Input: part model. Units: mm. Frame: model coordinates. A direction names the side the tool comes from. Coordinates: 2 decimals unless noted, no trailing zeros. Loops run counter-clockwise (first coordinate to the right, second up) from the corner with the lowest first, then second, coordinate; pieces in that order, holes last. Notation, with made-up numbers: (67, 2.5) -> (121, 2.5) arc R29 ccw to (121, 38.5) -> close; hole circle Ø8 at (-33.5, -5.5). An arc over 180 degrees is marked (long way). Answer as a JSON object with one key per item and string values.
from build123d import *

# Parameters (mm, degrees)
ESQUISSE1_R      = 21.5
EXTRUSION1_DEPTH = 30
ESQUISSE2_R      = 10
EXTRUSION2_DEPTH = 5
ESQUISSE3_R      = 4
EXTRUSION3_DEPTH = 20
ESQUISSE4_R      = 17
EXTRUSION4_DEPTH = 40
ESQUISSE5_R      = 4
EXTRUSION5_DEPTH = 1


with BuildPart() as part:
    # Esquisse1 → Extrusion1 (new body)
    with BuildSketch(Plane.XY):
        Circle(ESQUISSE1_R)
    extrude(amount=EXTRUSION1_DEPTH)

    # Esquisse2 → Extrusion2 (add)
    with BuildSketch(Plane.XY.offset(30)):
        Circle(ESQUISSE2_R)
    extrude(amount=EXTRUSION2_DEPTH)

    # Esquisse3 → Extrusion3 (add)
    with BuildSketch(Plane.XY.offset(35)):
        Circle(ESQUISSE3_R)
    extrude(amount=EXTRUSION3_DEPTH)

    # Esquisse4 → Extrusion4 (add)
    with BuildSketch(Plane(origin=(0, 0, 0), x_dir=(-1, 0, 0), z_dir=(0, 0, -1))):
        with Locations(Location((0, 0, 0), (0, 0, 180))):
            Circle(ESQUISSE4_R)
    extrude(amount=EXTRUSION4_DEPTH)

    # Esquisse5 → Extrusion5 (add)
    with BuildSketch(Plane.XY.offset(30)):
        with Locations(Location((0, 17.5, 0), (0, 0, 89.999550935))):
            Circle(ESQUISSE5_R)
        with Locations(Location((-15.155444566, -8.75, 0), (0, 0, 209.999550935))):
            Circle(ESQUISSE5_R)
        with Locations(Location((15.155444566, -8.75, 0), (0, 0, 329.999550935))):
            Circle(ESQUISSE5_R)
    extrude(amount=EXTRUSION5_DEPTH)


solid = part.part
1. Line query: line 1 along Z through (x, y) = (-11, 10.5); line 2 along Z through (x, y) = (11, -16.5); line 3 along Y through (x, z) = (-14, -32). Output: solid intervals per line, ascending.
Reply:
{"line 1": "z = -40 to 30", "line 2": "z = 0 to 30", "line 3": "y = -9.64 to 9.64"}
2. Section query A-A (y = 0). Return loops of the section in (x, z).
Reply:
{"outline": "(-21.5, 0) -> (-17, 0) -> (-17, -40) -> (17, -40) -> (17, 0) -> (21.5, 0) -> (21.5, 30) -> (10, 30) -> (10, 35) -> (4, 35) -> (4, 55) -> (-4, 55) -> (-4, 35) -> (-10, 35) -> (-10, 30) -> (-21.5, 30) -> close"}
3. Access query for faces 1 (the face through (-15, -9, 31)), 2 (the face through (4.5, -9.3, 30)), 3 (the face through (0, 17, 31)), 4 (the face through (-16, -6.3, 0)). Directions: +Z, -Z, +X, -X, +Y, -Y. A direction counts if a zero-diameter tool reaches every point of the face in a straight line with its end or side. Return the directions, or none.
Reply:
{"face 1": "+Z, -X, +Y, -Y", "face 2": "+Z", "face 3": "+Z, +X, -X, +Y", "face 4": "-Z"}
4. Section query B-B (x = 15). Return loops of the section in (y, z), plus the area to 3 significant figures.
Reply:
{"outline": "(-15.4, 0) -> (-8, 0) -> (-8, -40) -> (8, -40) -> (8, 0) -> (15.4, 0) -> (15.4, 30) -> (-4.75, 30) -> (-4.75, 31) -> (-12.75, 31) -> (-12.75, 30) -> (-15.4, 30) -> close", "area": "1,570 mm2"}
5. Mould query, pull axis X, two halves, no side actions, for faces 5 (the face through (-13.623, -5.055, 30.493)), 6 (the face through (15, -9, 31)), 7 (the face through (-2.213, -16.855, -19.72)). Classes: pulls with the +X half, pulls with the -X half, needs draft (parallel to the pull), parting line crosses it, or undercut.
Reply:
{"face 5": "undercut", "face 6": "needs draft", "face 7": "parting line crosses it"}
6. Section query D-D (y = -8.75). Return loops of the section in (x, z), plus the area to 3 significant figures.
Reply:
{"outline": "(-19.64, 0) -> (-14.58, 0) -> (-14.58, -40) -> (14.58, -40) -> (14.58, 0) -> (19.64, 0) -> (19.64, 30) -> (19.16, 30) -> (19.16, 31) -> (11.16, 31) -> (11.16, 30) -> (4.84, 30) -> (4.84, 35) -> (-4.84, 35) -> (-4.84, 30) -> (-11.16, 30) -> (-11.16, 31) -> (-19.16, 31) -> (-19.16, 30) -> (-19.64, 30) -> close", "area": "2,410 mm2"}
7. Section query C-C (z = 22.5). Return loops of the section in (x, y).
Reply:
{"outline": "circle Ø43 at (0, 0)"}
8. Pin query (flat end, axial travel): P1, Ø6.5, axis at x = 0.5, y = 19, coming from the +Z side; P2, Ø3, axis at y = 7.5, z = -29.5, coming from the +X side; P3, Ø4, axis at y = -2.5, z = -13, coming from the +X side. Return the tip coordinate at first contact, or that it passes through.
Reply:
{"P1": "stops at z = 31", "P2": "stops at x = 15.91", "P3": "stops at x = 16.99"}
